```python
from build123d import *

# Parameters (mm, degrees)
F0_R     = 37.5
F0_R_2   = 22
F1_DEPTH = 110
F2_SIZE  = 4
F3_SIZE  = 3
F4_R     = 2.5
F5_DEPTH = 38.5000001


with BuildPart() as f1:
    # F0 (on Top) → F1 (new body)
    with BuildSketch(Plane.XY):
        Circle(F0_R)
        Circle(F0_R_2, mode=Mode.SUBTRACT)
    extrude(amount=F1_DEPTH)

    # F2
    f2_edges = [f1.edges().sort_by_distance(p)[0] for p in [
        (-37.5, 0, 110),
        (-37.5, 0, 0),
    ]]
    chamfer(f2_edges, length=F2_SIZE)

    # F3
    f3_edges = [f1.edges().sort_by_distance(p)[0] for p in [
        (-22, 0, 110),
        (-22, 0, 0),
    ]]
    chamfer(f3_edges, length=F3_SIZE)

    # F4 (on Right) → F5 (cut, up to face)
    with BuildSketch(Plane.YZ):
        with Locations((0, 55)):
            Circle(F4_R)
    extrude(amount=F5_DEPTH, mode=Mode.SUBTRACT)


solid = f1.part
```
Can you work these out from the model? Positions are in its coordinate system, mm. Round coordinates to 2 decimals unless told otherwise and drop trailing zeros. Order: outer loops, then holes, each group sorted by start corner. A loop starts at its lowest first (then second) coordinate and runs counter-clockwise, first axis right, second up. Notation, with made-up numbers: (-12, -11.5) -> (8, -11.5) arc R35 cw to (8, 20.5) -> close; hole circle Ø11 at (-15, 36). An arc over 180 degrees is marked (long way). Return JSON: item names as keys, results as strings. Group by question number.
1. If we section it at C-C, the plane z = 18.5: Write out the boundary of the cut face in (x, y).
2. We'd pull the mould along Y, two halves only. Please class faces 1 (the face through (29.57, -0.54, 52.56)), 2 (the face through (-17.574, -13.475, 107.146)), 3 (the face through (-13, -22, 0)), 4 (the face through (31.12, -12.91, 0.19)): released by +Y, released by -Y, zero draft, split by the parting line, or undercut.
3. Will these pins go through, and if not, where does the flat tip stop? pin 1 (2 mm diameter, centred on x = 12, z = 63.5, fed in from +Y); pin 2 (3 mm diameter, centred on x = -19, y = 29.5, fed in from -Z); pin 3 (3 mm diameter, centred on y = 19.5, z = 93, fed in from -X).
4. If we section it at D-D, the plane z = 55: Write out the boundary of the cut face in (x, y).
5. If we section it at A-A, the plane y = 0: Write out the boundary of the cut face in (x, z), then the cut area to 3 significant figures.
6. If we section it at B-B, the plane x = 0: Write out the boundary of the cut face in (y, z).
7. I need wall thicknesses on line 1 (X direction, y = -2.5, z = 57); line 2 (X direction, y = 19, z = 104.5); line 3 (Y direction, x = 0, z = 79). Which ranges of each line are inside material? Lowest first, please. Write a range as [from, to].
Output values:
{
 "1": {"outline": "circle Ø75 at (0, 0); hole circle Ø44 at (0, 0)"},
 "2": {"face 1": "undercut", "face 2": "undercut", "face 3": "zero draft", "face 4": "split by the parting line"},
 "3": {"pin 1": "y = 35.85", "pin 2": "z = 0.09", "pin 3": "x = -32.9"},
 "4": {"outline": "(21.86, -2.5) arc R22 cw (long way) to (21.86, 2.5) -> (37.42, 2.5) arc R37.5 ccw (long way) to (37.42, -2.5) -> close"},
 "5": {"outline": "(-37.5, 4) -> (-33.5, 0) -> (-25, 0) -> (-22, 3) -> (-22, 107) -> (-25, 110) -> (-33.5, 110) -> (-37.5, 106) -> close; (22, 3) -> (25, 0) -> (33.5, 0) -> (37.5, 4) -> (37.5, 52.5) -> (22, 52.5) -> close; (22, 57.5) -> (37.5, 57.5) -> (37.5, 106) -> (33.5, 110) -> (25, 110) -> (22, 107) -> close", "area": "3,280 mm²"},
 "6": {"outline": "(-37.5, 4) -> (-33.5, 0) -> (-25, 0) -> (-22, 3) -> (-22, 107) -> (-25, 110) -> (-33.5, 110) -> (-37.5, 106) -> close; (22, 3) -> (25, 0) -> (33.5, 0) -> (37.5, 4) -> (37.5, 106) -> (33.5, 110) -> (25, 110) -> (22, 107) -> close"},
 "7": {"line 1": "[-37.42, -21.86], [21.86, 37.42]", "line 2": "[-32.33, -11.09], [11.09, 32.33]", "line 3": "[-37.5, -22], [22, 37.5]"}
}
